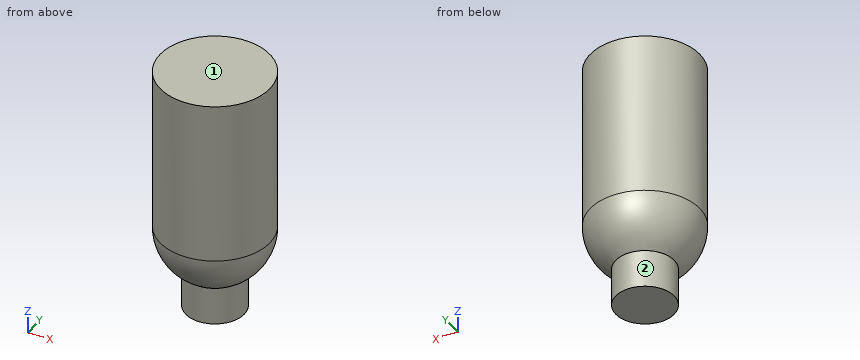
```python
from build123d import *

# Parameters (mm, degrees)
F1_ANGLE = -180
F2_R     = 152.4
F3_DEPTH = 438.15
F4_R     = 285.75
F5_DEPTH = 850.9


with BuildPart() as f1:
    # F0 (on Top) → F1 (revolve)
    with BuildSketch(Plane.XY):
        with BuildLine():
            Line((0, 0), (285.75, 0))
            ThreePointArc((285.75, 0), (0, 285.75), (-285.75, 0))
            Line((-285.75, 0), (0, 0))
        make_face()
    revolve(axis=Axis((142.875, 0, 0), (1, 0, 0)), revolution_arc=F1_ANGLE)

    # F2 (on face) → F3 (join)
    with BuildSketch(Plane.XY):
        Circle(F2_R)
    extrude(amount=-F3_DEPTH)

    # F4 (on face) → F5 (join)
    with BuildSketch(Plane.XY):
        Circle(F4_R)
    extrude(amount=F5_DEPTH)


solid = f1.part
```
Check sheet for the modelled part. Datum: model origin and axes. Units: mm. Face numbers are marked on the shaded views. A direction names the side the tool comes from. Give positions to 0.01 mm unless a question says otherwise; leave off trailing zeros. Loops run counter-clockwise (first coordinate to the right, second up) from the corner with the lowest first, then second, coordinate; pieces in that order, holes last. Notation, with made-up numbers: (-7.75, -16.5) - (50.25, -16.5) arc R21 cw to (50.25, 7.5) - close; hole circle Ø8 at (-15.5, -9). An arc over 180 degrees is marked (long way). One line per question, with ' | ' between items. Start each with the question number.
1. Cross-section at C-C, the plane z = -264.5. Enter the section's corners in (x, y).
2. Set-up check for the marked faces 1 and 2: record each of +Z, -Z, +X, -X, +Y, -Y from which the full face is reachable in a straight line by a thin tool's end or side.
3. Gauge pin test, flat ends, axial feed: pin 1 Ø12 at (x, y) = (-111, 169) entering from -Z; pin 2 Ø3 at (x, z) = (-24.5, -132.5) entering from -Y; pin 3 Ø2 at (x, z) = (64, 184.5) entering from +Y. Record the tip position at first contact, or that the pin passes through.
4. Cross-section at D-D, the plane z = 171. Enter the section's corners in (x, y), plus the area to 3 significant figures.
5. Cross-section at A-A, the plane y = 0. Enter the section's corners in (x, z).
6. Material ranges on line 1 along Y through (x, z) = (215.5, -24); line 2 along Y through (x, z) = (156, -180.5); line 3 along Z through (x, y) = (-26, -208), recorded low to high. Write a range as [from, to].
Check result:
1) outline: circle Ø304.8 at (0, 0)
2) face 1: +Z, +X, -X, +Y, -Y | face 2: -Z
3) pin 1: stops at z = -207.75 | pin 2: stops at y = -252.78 | pin 3: stops at y = 278.72
4) outline: circle Ø571.5 at (0, 0) | area: 257,000 mm2
5) outline: (-285.75, 0) arc R285.75 ccw to (-152.4, -241.72) - (-152.4, -438.15) - (152.4, -438.15) - (152.4, -241.72) arc R285.75 ccw to (285.75, 0) - (285.75, 850.9) - (-285.75, 850.9) - close
6) line 1: y = [-186.11, 186.11] | line 2: y = [-157.28, 157.28] | line 3: z = [-194.2, 850.9]
